Part model, mm, in its own coordinate system. A direction names the side the tool comes from. Coordinates: 2 decimals unless noted, no trailing zeros. Loops run counter-clockwise (first coordinate to the right, second up) from the corner with the lowest first, then second, coordinate; pieces in that order, holes last. Notation, with made-up numbers: M -21,36 L 19,36 A13 cw 19,40 Z; hole C 28.5,72 d2. An arc over 180 degrees is marked long. Use a Markdown table: item, result. Add a question column.
1) Band-saw the part on B-B (y = 51). List the corners of the cut face in (x, z) (3 decimals).
2) Tool access for faces 5 (the flat face through (22.871, 19, 28)), 6 (the cylindrical face through (-39.747, -35.24, 20.776)), 7 (the flat face through (102, -1, 38.952)): list every direction of +Z, -Z, +X, -X, +Y, -Y with a clear straight run to the whole face (end or side of a thin tool).
3) Wall check: probe 1 along Y at (x, z) = (37, 24); probe 2 along X at (y, z) = (-33, -10.5) (3 decimals); probe 3 along Z at (x, y) = (18.5, 35) (3 decimals). Give the ranges that are in metal, low to high. Write a range as from..to.
4) Pin check, flat tips, straight feed: pin 1 Ø23 at (x, y) = (-16, -37.5) entering from +Z (3 decimals); pin 2 Ø1 at (x, z) = (103.5, 41.5) entering from +Y; pin 3 Ø10 at (x, z) = (92, 53) entering from +Y. Stop position of each tip, or through.
5) Pull direction X, two halves, no side cores. Call faces 1 (the cylindrical face through (45.766, -0.356, 45.19)), 2 (the cylindrical face through (-0.51, 61.97, 20.78)), 3 (the cylindrical face through (-39.747, 35.88, 20.776)), 4 (the cylindrical face through (101.984, 18.784, 42.126)): released by +X, released by -X, zero draft, split by the parting line, or undercut.
6) Band-saw the part on A-A (z = -2). List the corners of the cut face in (x, y) (3 decimals).
from build123d import *

# Parameters (mm, degrees)
F1_DEPTH = 63.5
F2_DEPTH = 12.7
F0_W     = 37.7701045194
F0_H     = 18.4038491807
F3_DEPTH = 25.4
F0_W_2   = 38.1
F0_H_2   = 38.1
F5_R     = 5.08
F6_D     = 6.35
F6_DEPTH = 63.501


with BuildPart() as f1:
    # F0 (on Front) → F1 (new body, symmetric)
    with BuildSketch(Plane.XZ):
        Polygon((22.8711508193, 22.2250013784), (-41.275, 22.2250013784), (-41.275, -22.2250013784), (41.275, -22.2250013784), (41.275, 22.2250013784), align=None)
    extrude(amount=F1_DEPTH, both=True)

    # F0 (on Front) → F2 (join, symmetric)
    with BuildSketch(Plane.XZ):
        with BuildLine():
            add(Edge.make_bspline(
                [(-41.275, 22.2250013784), (-39.927624166, 47.3601222038), (-12.1371774003, 68.6116442084), (57.023, 68.3297926274)],
                knots=[0, 0, 0, 0, 108.5732406264, 108.5732406264, 108.5732406264, 108.5732406264], degree=3))
            Line((-41.275, 22.2250013784), (22.8711508193, 22.2250013784))
            Line((22.8711508193, 22.2250013784), (22.8711508193, 34.1779434467))
            ThreePointArc((22.8711508193, 34.1779434467), (32.8739958543, 58.3269475924), (57.023, 68.3297926274))
        make_face()
    extrude(amount=F2_DEPTH, both=True)

    # F0 (on Front) → F3 (join, symmetric)
    with BuildSketch(Plane.XZ):
        with BuildLine():
            Line((22.8711508193, 34.1779434467), (22.8711508193, 22.2250013784))
            Line((22.8711508193, 22.2250013784), (41.275, 22.2250013784))
            Line((41.275, 22.2250013784), (41.275, 34.1779434467))
            ThreePointArc((41.275, 34.1779434467), (45.8874824099, 45.3134610369), (57.023, 49.9259434467))
            Line((57.023, 49.9259434467), (63.813790679, 49.9259434467))
            Line((63.813790679, 49.9259434467), (63.813790679, 68.3297926274))
            Line((63.813790679, 68.3297926274), (57.023, 68.3297926274))
            ThreePointArc((57.023, 68.3297926274), (32.8739958543, 58.3269475924), (22.8711508193, 34.1779434467))
        make_face()
        with Locations((82.6988429387, 59.1278680371)):
            Rectangle(F0_W, F0_H)
    extrude(amount=F3_DEPTH, both=True)

    # F0 (on Front) → F4 (revolve)
    with BuildSketch(Plane.XZ):
        with Locations((120.963790679, 58.0022351325)):
            Rectangle(F0_W_2, F0_H_2)
    revolve(axis=Axis((101.913790679, 0, 58.0022351325), (0, 0, -1)))

    # F5
    f5_edges = [f1.edges().sort_by_distance(p)[0] for p in [
        (41.275, -63.5, 0),
        (41.275, 63.5, 0),
        (-41.275, 63.5, 0),
        (-41.275, -63.5, 0),
        (0, -63.5, 22.225001),
        (-41.275, -38.1, 22.225001),
        (-41.275, 38.1, 22.225001),
        (41.275, -44.45, 22.225001),
        (41.275, 44.45, 22.225001),
        (0, 63.5, 22.225001),
    ]]
    fillet(f5_edges, radius=F5_R)

    # F6 (through all, one way)
    with BuildSketch(Plane.XZ):
        with Locations((101.913790679, 77.0522351325), (101.913790679, 38.9522351325)):
            Circle(F6_D / 2)
    extrude(amount=-F6_DEPTH, mode=Mode.SUBTRACT)


solid = f1.part
Entries:
| question | item | result |
|---|---|---|
| 1 | outline | M -41.275,-22.225 L 41.275,-22.225 L 41.275,17.145 A5.08 ccw 36.195,22.225 L -36.195,22.225 A5.08 ccw -41.275,17.145 Z |
| 2 | face 5 | +Z, -X, +Y |
| 2 | face 6 | +Z, -X, -Y |
| 2 | face 7 | -Z, +X, +Y, -Y |
| 3 | probe 1 | -25.4..25.4 |
| 3 | probe 2 | -41.275..41.275 |
| 3 | probe 3 | -22.225..22.225 |
| 4 | pin 1 | z = 22.225 |
| 4 | pin 2 | y = 38.08 |
| 4 | pin 3 | y = 37.78 |
| 5 | face 1 | undercut |
| 5 | face 2 | zero draft |
| 5 | face 3 | released by -X |
| 5 | face 4 | undercut |
| 6 | outline | M -41.275,-58.42 A5.08 ccw -36.195,-63.5 L 36.195,-63.5 A5.08 ccw 41.275,-58.42 L 41.275,58.42 A5.08 ccw 36.195,63.5 L -36.195,63.5 A5.08 ccw -41.275,58.42 Z |
